Here's how the part is built. I have some questions about the finished solid (model axes, mm). A direction names the side the tool comes from. Round coordinates to 2 decimals unless told otherwise and drop trailing zeros. Write each loop counter-clockwise with the first axis right and the second up, starting at its lowest first coordinate (ties: lowest second). Pieces come first, ordered by that corner, then holes. Notation, with made-up numbers: M -4.75,53.5 L 22.25,53.5 A26 cw 22.25,82.5 Z; hole C 17.25,21 d6. An arc over 180 degrees is marked long. Use one line per item in the form item = value. Start each with the question number.
Q1. I want a section at A-A on z = 206.5. List the corners of the cut face in (x, y) for me, and give its area (3 significant figures).
Q2. We'd pull the mould along X, two halves only. Please class faces 1 (the face through (-30, -500, 129)), 2 (the face through (477.134, -7, 129)), 3 (the face through (9, -640, 158)), 4 (the face through (-640, -9, 158)): +X half, -X half, draft (parallel to the pull), parting line (faces both ways), or undercut.
Q3. For faces 5 (the face through (625, -9, 170)), 6 (the face through (640, -9, 162)), which set-ups out of +Z, -Z, +X, -X, +Y, -Y let a thin tool reach every point of the face, with its end or its side?
Q4. I want a section at C-C on x = 562. List the corners of the cut face in (y, z) for me.
Q5. I'm going to push a flat-ended pin straight in: pin 1 Ø12 at (x, y) = (-355.5, 468) entering from +Z. Where does the tip first touch, or does it pass through?
Q6. I need wall thicknesses on line 1 along Y through (x, z) = (-397, 236); line 2 along X through (y, z) = (46, 162); line 3 along Y through (x, z) = (233, 248). Which ranges of each line are inside material? Lowest first, please. Write a range as from..to.
Q7. I want a section at B-B on y = -168. List the corners of the cut face in (x, z) for me.
```python
from build123d import *

# Parameters (mm, degrees)
F0_W      = 1250
F0_H      = 1250
F1_DEPTH  = 15
F2_W      = 1265
F2_H      = 320
F6_DEPTH  = 15
F3_W      = 1265
F3_H      = 320
F7_DEPTH  = 15
F4_W      = 1265
F4_H      = 320
F8_DEPTH  = 15
F5_W      = 1265
F5_H      = 320
F9_DEPTH  = 15
F11_W     = 1000
F11_H     = 1000
F12_DEPTH = 231


with BuildPart() as f1:
    # F0 (on Top) → F1 (new body)
    with BuildSketch(Plane.XY):
        Rectangle(F0_W, F0_H)
    extrude(amount=F1_DEPTH)

    # F2 (on face) → F6 (join)
    with BuildSketch(Plane.XZ.offset(625)):
        with Locations((7.5, 160)):
            Rectangle(F2_W, F2_H)
    extrude(amount=F6_DEPTH)

    # F3 (on face) → F7 (join)
    with BuildSketch(Plane.YZ.offset(625)):
        with Locations((7.5, 160)):
            Rectangle(F3_W, F3_H)
    extrude(amount=F7_DEPTH)

    # F4 (on face) → F8 (join)
    with BuildSketch(Plane(origin=(-625, 0, 0), x_dir=(0, -1, 0), z_dir=(-1, 0, 0))):
        with Locations((7.5, 160)):
            Rectangle(F4_W, F4_H)
    extrude(amount=F8_DEPTH)

    # F5 (on face) → F9 (join)
    with BuildSketch(Plane(origin=(0, 625, 0), x_dir=(-1, 0, 0), z_dir=(0, 1, 0))):
        with Locations((7.5, 160)):
            Rectangle(F5_W, F5_H)
    extrude(amount=F9_DEPTH)

    # F11 (on face) → F12 (join)
    with BuildSketch(Plane.XY.offset(15)):
        with Locations((-22.866359, 0)):
            Rectangle(F11_W, F11_H)
    extrude(amount=F12_DEPTH)


solid = f1.part
```
Reported:
q1.outline = M -640,-640 L 640,-640 L 640,640 L -640,640 Z; M -522.87,-500 L 477.13,-500 L 477.13,500 L -522.87,500 Z; hole M -625,-625 L 625,-625 L 625,625 L -625,625 Z
q1.area = 1,080,000 mm^2
q2.face_1 = undercut
q2.face_2 = undercut
q2.face_3 = draft
q2.face_4 = -X half
q3.face_5 = +Z
q3.face_6 = +Z, -Z, +X, +Y, -Y
q4.outline = M -640,0 L 640,0 L 640,320 L 625,320 L 625,15 L -625,15 L -625,320 L -640,320 Z
q5.pin_1 = 246
q6.line_1 = -640..-625, -500..500, 625..640
q6.line_2 = -640..-625, -522.87..477.13, 625..640
q6.line_3 = -640..-625, 625..640
q7.outline = M -640,0 L 640,0 L 640,320 L 625,320 L 625,15 L 477.13,15 L 477.13,246 L -522.87,246 L -522.87,15 L -625,15 L -625,320 L -640,320 Z
